```python
from build123d import *

# Parameters (mm, degrees)
F0_W     = 6.35
F0_H     = 66.675
F1_DEPTH = 165.1
F2_R     = 41.275


with BuildPart() as f1:
    # F0 (on Top) → F1 (new body)
    with BuildSketch(Plane.XY):
        with BuildLine():
            Line((31.75, 0), (38.1, 0))
            ThreePointArc((38.1, 0), (0, 38.1), (-38.1, 0))
            Line((-38.1, 0), (-31.75, 0))
            ThreePointArc((-31.75, 0), (0, 31.75), (31.75, 0))
        make_face()
        with Locations((-34.925, -33.3375)):
            Rectangle(F0_W, F0_H)
        with Locations((34.925, -33.3375)):
            Rectangle(F0_W, F0_H)
    extrude(amount=F1_DEPTH)

    # F2
    f2_edges = [f1.edges().sort_by_distance(p)[0] for p in [
        (-34.925, -66.675, 165.1),
        (34.925, -66.675, 165.1),
        (-34.925, -66.675, 0),
        (34.925, -66.675, 0),
    ]]
    fillet(f2_edges, radius=F2_R)


solid = f1.part
```
Design review of the part built by this model. Coordinates are the model's own, in mm. A direction names the side the tool comes from. Round coordinates to 2 decimals unless told otherwise and drop trailing zeros. Write each loop counter-clockwise with the first axis right and the second up, starting at its lowest first coordinate (ties: lowest second). Pieces come first, ordered by that corner, then holes. Notation, with made-up numbers: (-36, 57.25) -> (17, 57.25) arc R7 cw to (17, 70.25) -> close; hole circle Ø1 at (34.5, 25.25). An arc over 180 degrees is marked (long way). Write item = value, one per line. Start each with the question number.
1) Clearance check with flat-ended pins moving along their axes: pin 1 (8 mm diameter, centred on x = -28, z = 53, fed in from -Y) (3 decimals); pin 2 (2 mm diameter, centred on x = 30, y = -13, fed in from -Z); pin 3 (5 mm diameter, centred on y = 22.5, z = 48.5, fed in from -X); pin 4 (4 mm diameter, centred on x = -30, z = 48.5, fed in from +Y). State where each tip first meets the part, or that it passes through.
2) Tool access review of faces 5 (the face through (-34.881, -54.905, 12.412)), 6 (the face through (-31.75, -34, 81)): name each direction out of +Z, -Z, +X, -X, +Y, -Y from which nothing blocks a thin tool from reaching the whole face with its end or side.
3) Take a section at C-C, the plane x = 19.5. State the section outline as (y, z) points.
4) Take a section at B-B, the plane y = 5.5. State the section outline as (x, z) points.
5) Take a section at D-D, the plane z = 154. State the section outline as (x, y) points, plus the area to 3 significant figures.
6) Mouldability with a two-part tool opening along X and no side actions: class faces 1 (the face through (38.1, -34, 81)), 2 (the face through (-38.1, -34, 81)), 3 (the face through (34.969, -54.905, 152.688)), 4 (the face through (-0.698, 31.742, 81.394)) as +X half, -X half, draft (parallel to the pull), parting line (faces both ways), or undercut.
7) Wall thickness on probe 1 along X at (y, z) = (-13, 83); probe 2 along Y at (x, z) = (-1, 99): over which ranges is each line inside the solid? List them lowest first. Write a range as from..to.
8) Take a section at A-A, the plane z = 57. State the section outline as (x, y) points (3 decimals).
Results list:
q1.pin_1 = -66.675
q1.pin_2 = through
q1.pin_3 = -32.43
q1.pin_4 = 25.84
q2.face_5 = -Z, +X, -X, -Y
q2.face_6 = +Z, -Z, -Y
q3.outline = (25.06, 0) -> (32.73, 0) -> (32.73, 165.1) -> (25.06, 165.1) -> close
q4.outline = (-37.7, 0) -> (-31.27, 0) -> (-31.27, 165.1) -> (-37.7, 165.1) -> close; (31.27, 0) -> (37.7, 0) -> (37.7, 165.1) -> (31.27, 165.1) -> close
q5.outline = (-38.1, -53.56) -> (-31.75, -53.56) -> (-31.75, 0) arc R31.75 cw to (31.75, 0) -> (31.75, -53.56) -> (38.1, -53.56) -> (38.1, 0) arc R38.1 ccw to (-38.1, 0) -> close
q5.area = 1,380 mm²
q6.face_1 = +X half
q6.face_2 = -X half
q6.face_3 = draft
q6.face_4 = undercut
q7.probe_1 = -38.1..-31.75, 31.75..38.1
q7.probe_2 = 31.73..38.09
q8.outline = (-38.1, -66.675) -> (-31.75, -66.675) -> (-31.75, 0) arc R31.75 cw to (31.75, 0) -> (31.75, -66.675) -> (38.1, -66.675) -> (38.1, 0) arc R38.1 ccw to (-38.1, 0) -> close
